Can you work these out from the model? Positions are in its coordinate system, mm. A direction names the side the tool comes from. Coordinates: 2 decimals unless noted, no trailing zeros. Order: outer loops, then holes, each group sorted by start corner. A loop starts at its lowest first (then second) coordinate and runs counter-clockwise, first axis right, second up. Notation, with made-up numbers: (-21, 69.25) -> (-6, 69.25) arc R16 cw to (-6, 82.25) -> close; hole circle Ø10 at (51.5, 24.5). An arc over 180 degrees is marked (long way). Write item = value, one per line.
```python
from build123d import *

# Parameters (mm, degrees)
SKETCH1_W           = 137.16
SKETCH1_H           = 87.122
SKETCH1_R           = 1.397
BOSS_EXTRUDE1_DEPTH = 1.651
SKETCH2_W           = 14.732
SKETCH2_H           = 14.5288
BOSS_EXTRUDE2_DEPTH = 1.905
SKETCH3_W           = 17.018
SKETCH3_H           = 17.018
BOSS_EXTRUDE3_DEPTH = 1.524


with BuildPart() as part:
    # Sketch1 → Boss-Extrude1 (new body)
    with BuildSketch(Plane(origin=(0, 0, 0), x_dir=(1, 0, 0), z_dir=(0, 1, 0))):
        with Locations((-68.58, 43.561)):
            Rectangle(SKETCH1_W, SKETCH1_H)
        with Locations(Location((-133.35, 83.312, 0), (0, 0, 90))):
            Circle(SKETCH1_R, mode=Mode.SUBTRACT)
        with Locations(Location((-3.81, 3.81, 0), (0, 0, 90))):
            Circle(SKETCH1_R, mode=Mode.SUBTRACT)
        with Locations(Location((-3.81, 83.312, 0), (0, 0, 90))):
            Circle(SKETCH1_R, mode=Mode.SUBTRACT)
        with Locations(Location((-133.35, 3.81, 0), (0, 0, 90))):
            Circle(SKETCH1_R, mode=Mode.SUBTRACT)
    extrude(amount=BOSS_EXTRUDE1_DEPTH)

    # Sketch2 → Boss-Extrude2 (add)
    with BuildSketch(Plane.XZ):
        with Locations((-57.404, -4.4704)):
            Rectangle(SKETCH2_W, SKETCH2_H)
    extrude(amount=BOSS_EXTRUDE2_DEPTH)

    # Sketch3 → Boss-Extrude3 (add)
    with BuildSketch(Plane(origin=(0, 1.651, 0), x_dir=(1, 0, 0), z_dir=(0, 1, 0))):
        with Locations((-82.169, 45.466)):
            Rectangle(SKETCH3_W, SKETCH3_H)
    extrude(amount=BOSS_EXTRUDE3_DEPTH)


solid = part.part
```
Item 1: I'm going to push flat-ended pins straight in: P1, Ø1.2, axis at x = -83.5, y = 2.5, coming from the -Z side (3 decimals); P2, Ø12, axis at x = -33, z = -7.5, coming from the +Y side; P3, Ø0.8, axis at x = -61.5, y = 1, coming from the +Z side; P4, Ø2.5, axis at x = -3.81, z = -83.312, coming from the -Y side. Where does each tip first touch, or does it pass through?
A:
P1 = -53.975
P2 = 1.65
P3 = 0
P4 = through
Item 2: I want a section at D-D, the plane z = -47. Please give me the cut outline in (x, y) (3 decimals), plus the area to 3 significant figures.
A:
outline = (-137.16, 0) -> (0, 0) -> (0, 1.651) -> (-73.66, 1.651) -> (-73.66, 3.175) -> (-90.678, 3.175) -> (-90.678, 1.651) -> (-137.16, 1.651) -> close
area = 252 mm2
Item 3: For faces 1 (the flat face through (-58, 0, 1)), 2 (the cylindrical face through (-134.735, 0.814, -83.13)), which set-ups out of +Z, -Z, +X, -X, +Y, -Y let a thin tool reach every point of the face, with its end or its side?
A:
face_1 = +Z, +X, -X, +Y
face_2 = +Y, -Y
Item 4: I want a section at A-A, the plane z = -3.81. Please give me the cut outline in (x, y) (3 decimals).
A:
outline = (-137.16, 0) -> (-134.747, 0) -> (-134.747, 1.651) -> (-137.16, 1.651) -> close; (-131.953, 0) -> (-64.77, 0) -> (-64.77, -1.905) -> (-50.038, -1.905) -> (-50.038, 0) -> (-5.207, 0) -> (-5.207, 1.651) -> (-131.953, 1.651) -> close; (-2.413, 0) -> (0, 0) -> (0, 1.651) -> (-2.413, 1.651) -> close
Item 5: I want a section at C-C, the plane x = -63. Please give me the cut outline in (y, z) (3 decimals).
A:
outline = (-1.905, -11.735) -> (0, -11.735) -> (0, -87.122) -> (1.651, -87.122) -> (1.651, 0) -> (0, 0) -> (0, 2.794) -> (-1.905, 2.794) -> close
Item 6: If we mould it in two halves opening along Z, with no side actions, what happens to faces 3 (the cylindrical face through (-2.57, 0.81, -4.45)), 4 (the flat face through (-58, -1.905, -4))? For each: pulls with the +Z half, pulls with the -Z half, needs draft (parallel to the pull), parting line crosses it, or undercut.
A:
face_3 = undercut
face_4 = needs draft
Item 7: If I drill on probe 1 along X at (y, z) = (0.75, -3.81); probe 2 along Z at (x, y) = (-133.35, 0.9) (3 decimals); probe 3 along X at (y, z) = (3, -37.5), over which ranges is the centre line in solid material (lowest first)?
A:
probe_1 = -137.16 to -134.75, -131.95 to -5.21, -2.41 to 0
probe_2 = -87.122 to -84.709, -81.915 to -5.207, -2.413 to 0
probe_3 = -90.68 to -73.66
Item 8: I want a section at B-B, the plane x = -3.81. Please give me the cut outline in (y, z) (3 decimals).
A:
outline = (0, -87.122) -> (1.651, -87.122) -> (1.651, -84.709) -> (0, -84.709) -> close; (0, -81.915) -> (1.651, -81.915) -> (1.651, -5.207) -> (0, -5.207) -> close; (0, -2.413) -> (1.651, -2.413) -> (1.651, 0) -> (0, 0) -> close
